from build123d import *

# Parameters (mm, degrees)
F0_W     = 19.05
F0_H     = 6.35
F1_DEPTH = 3.81
F2_T     = -0.635
F4_DEPTH = 3.175
F5_W     = 1.27
F5_H     = 1.27
F6_DEPTH = 0.635


with BuildPart() as f1:
    # F0 (on Top) → F1 (new body)
    with BuildSketch(Plane.XY):
        with Locations((19.5798018083, 32.579488121)):
            Rectangle(F0_W, F0_H)
    extrude(amount=F1_DEPTH)

    # F2
    f2_openings = [f1.faces().sort_by_distance(p)[0] for p in [
        (19.579802, 32.579488, 3.81),
    ]]
    offset(amount=F2_T, openings=f2_openings)

    # F3 (on face) → F4 (join)
    with BuildSketch(Plane.XY.offset(0.635)):
        with BuildLine():
            ThreePointArc((22.9725916315, 35.119488121), (24.4037620723, 33.6883176802), (25.8349325131, 35.119488121))
            Line((25.8349325131, 35.119488121), (22.9725916315, 35.119488121))
        make_face()
    extrude(amount=F4_DEPTH)

    # F5 (on face) → F6 (cut)
    with BuildSketch(Plane(origin=(10.0548018083, 0, 0), x_dir=(0, -1, 0), z_dir=(-1, 0, 0))):
        with Locations((-33.214488121, 2.8575)):
            Rectangle(F5_W, F5_H)
        with Locations((-31.944488121, 2.8575)):
            Rectangle(F5_W, F5_H)
        with Locations((-31.944488121, 1.5875)):
            Rectangle(F5_W, F5_H)
        with Locations((-33.214488121, 1.5875)):
            Rectangle(F5_W, F5_H)
    extrude(amount=-F6_DEPTH, mode=Mode.SUBTRACT)


solid = f1.part
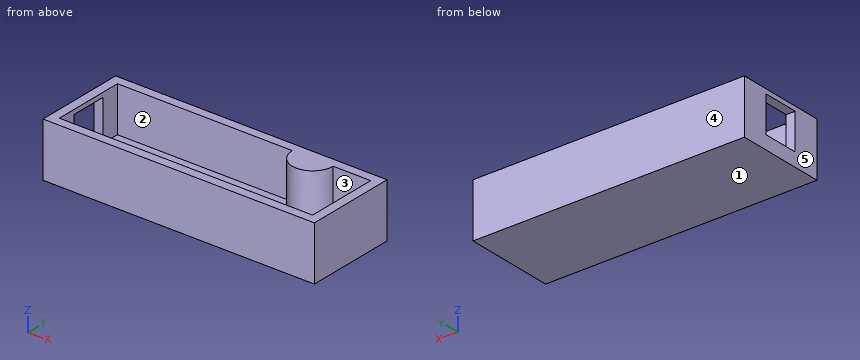
Could you check a few things on this model? Use its own coordinates, in mm. Face numbers are marked on the shaded views. A direction names the side the tool comes from. Coordinates: 2 decimals unless noted, no trailing zeros. Order: outer loops, then holes, each group sorted by start corner. A loop starts at its lowest first (then second) coordinate and runs counter-clockwise, first axis right, second up. Notation, with made-up numbers: (9, 27) - (35, 27) arc R27 ccw to (35, 51) - close; hole circle Ø9 at (83.25, 41). An arc over 180 degrees is marked (long way). Answer in a Markdown table with one row per item. Add a question column.
(1) If we section it at C-C, the plane x = 25.5: Please give me the cut outline in (y, z) (3 decimals), then the cut area to 3 significant figures.
(2) On a 3-axis mill with a long thin cutter (end or side, diameter ignored), from which of +Z, -Z, +X, -X, +Y, -Y can I reach the whole of each face in a straight line? I mean the marked faces 1 and 2. Say none if no direction works.
(3) I need wall thicknesses on L1, parallel to X at y = 33, z = 0.9; L2, parallel to X at y = 34, z = 2.8; L3, parallel to Y at x = 14.25, z = 3.65. Which ranges of each line are inside material? Lowest first, please.
(4) If we section it at B-B, the plane z = 1.3: Please give me the cut outline in (x, y), then the cut area to 3 significant figures.
(5) If we section it at D-D, the plane y = 30.25: Please give me the cut outline in (x, z) (3 decimals).
(6) If we mould it in two halves opening along X, with no side actions, what happens to the marked faces 3, 4 and 5? For each: released by +X, released by -X, zero draft, split by the parting line, or undercut.
Results are:
| question | item | result |
|---|---|---|
| 1 | outline | (29.404, 0) - (35.754, 0) - (35.754, 3.81) - (34.199, 3.81) - (34.199, 0.635) - (30.039, 0.635) - (30.039, 3.81) - (29.404, 3.81) - close |
| 1 | area | 11.0 mm2 |
| 2 | face 1 | -Z, +X, -X, +Y, -Y |
| 2 | face 2 | +Z |
| 3 | L1 | x = 10.05 to 10.69, 28.47 to 29.1 |
| 3 | L2 | x = 10.05 to 10.69, 23.51 to 25.3, 28.47 to 29.1 |
| 3 | L3 | y = 29.4 to 30.04, 35.12 to 35.75 |
| 4 | outline | (10.05, 29.4) - (29.1, 29.4) - (29.1, 35.75) - (10.05, 35.75) - (10.05, 33.85) - (10.69, 33.85) - (10.69, 35.12) - (22.97, 35.12) arc R1.43 ccw to (25.83, 35.12) - (28.47, 35.12) - (28.47, 30.04) - (10.69, 30.04) - (10.69, 31.31) - (10.05, 31.31) - close |
| 4 | area | 32.2 mm2 |
| 5 | outline | (10.055, 0) - (29.105, 0) - (29.105, 3.81) - (28.47, 3.81) - (28.47, 0.635) - (10.69, 0.635) - (10.69, 3.81) - (10.055, 3.81) - close |
| 6 | face 3 | undercut |
| 6 | face 4 | zero draft |
| 6 | face 5 | released by -X |
